```python
from build123d import *

# Parameters (mm, degrees)
SKETCH_1_W          = 104
SKETCH_1_H          = 52
SKETCH_1_R          = 11.25
EXTRUDE_1_DEPTH     = 6
SKETCH_2_R          = 2.15
SKETCH_2_R_2        = 5
CUT_EXTRUDE_1_DEPTH = 10
FILLET_2_R          = 5
SKETCH_3_R          = 1.6
SKETCH_3_R_2        = 2.1
CUT_EXTRUDE_2_DEPTH = 10
SKETCH1_R           = 4
CUT_EXTRUDE1_DEPTH  = 2


with BuildPart() as part:
    # 草图1 → 凸台-拉伸1 (new body)
    with BuildSketch(Plane(origin=(0, 0, 0), x_dir=(0, 0, -1), z_dir=(1, 0, 0))):
        with Locations((245.135135135, 41.033128111)):
            Rectangle(SKETCH_1_W, SKETCH_1_H)
        with Locations((220.135135135, 41.033128111)):
            Circle(SKETCH_1_R, mode=Mode.SUBTRACT)
        with Locations((270.135135135, 41.033128111)):
            Circle(SKETCH_1_R, mode=Mode.SUBTRACT)
    extrude(amount=EXTRUDE_1_DEPTH)

    # 草图2 → 切除-拉伸1 (cut)
    # profile 1 of 12: a face of its own
    with BuildSketch(Plane(origin=(6, 0, 0), x_dir=(0, 0, -1), z_dir=(1, 0, 0))):
        with Locations((198.135135135, 62.033128111)):
            Circle(SKETCH_2_R)
    # profile 2 of 12: a face of its own
    with BuildSketch(Plane(origin=(6, 0, 0), x_dir=(0, 0, -1), z_dir=(1, 0, 0))):
        with Locations((198.135135135, 20.033128111)):
            Circle(SKETCH_2_R)
    # profile 3 of 12: a face of its own
    with BuildSketch(Plane(origin=(6, 0, 0), x_dir=(0, 0, -1), z_dir=(1, 0, 0))):
        with Locations((245.135135135, 20.033128111)):
            Circle(SKETCH_2_R_2)
        with Locations((245.135135135, 20.033128111)):
            Circle(SKETCH_2_R, mode=Mode.SUBTRACT)
    # profile 4 of 12: a face of its own
    with BuildSketch(Plane(origin=(6, 0, 0), x_dir=(0, 0, -1), z_dir=(1, 0, 0))):
        with BuildLine():
            Line((245.13513516, 15.033128111), (250.135135135, 15.033128111))
            Line((250.135135135, 15.033128111), (250.135135135, 20.033128111))
            ThreePointArc((250.135135135, 20.033128111), (248.67066905, 16.497594214), (245.13513516, 15.033128111))
        make_face()
    # profile 5 of 12: a face of its own
    with BuildSketch(Plane(origin=(6, 0, 0), x_dir=(0, 0, -1), z_dir=(1, 0, 0))):
        with BuildLine():
            Line((240.135135135, 15.033128111), (245.13513516, 15.033128111))
            ThreePointArc((245.13513516, 15.033128111), (241.599601238, 16.497594196), (240.135135135, 20.033128111))
            Line((240.135135135, 20.033128111), (240.135135135, 15.033128111))
        make_face()
    # profile 6 of 12: a face of its own
    with BuildSketch(Plane(origin=(6, 0, 0), x_dir=(0, 0, -1), z_dir=(1, 0, 0))):
        with Locations((245.135135135, 20.033128111)):
            Circle(SKETCH_2_R)
    # profile 7 of 12: a face of its own
    with BuildSketch(Plane(origin=(6, 0, 0), x_dir=(0, 0, -1), z_dir=(1, 0, 0))):
        with Locations((245.135135135, 62.033128111)):
            Circle(SKETCH_2_R_2)
        with Locations((245.135135135, 62.033128111)):
            Circle(SKETCH_2_R, mode=Mode.SUBTRACT)
    # profile 8 of 12: a face of its own
    with BuildSketch(Plane(origin=(6, 0, 0), x_dir=(0, 0, -1), z_dir=(1, 0, 0))):
        with Locations((245.135135135, 62.033128111)):
            Circle(SKETCH_2_R)
    # profile 9 of 12: a face of its own
    with BuildSketch(Plane(origin=(6, 0, 0), x_dir=(0, 0, -1), z_dir=(1, 0, 0))):
        with BuildLine():
            ThreePointArc((245.135135095, 67.033128111), (248.670669027, 65.568662031), (250.135135135, 62.033128111))
            Line((250.135135135, 62.033128111), (250.135135135, 67.033128111))
            Line((250.135135135, 67.033128111), (245.135135095, 67.033128111))
        make_face()
    # profile 10 of 12: a face of its own
    with BuildSketch(Plane(origin=(6, 0, 0), x_dir=(0, 0, -1), z_dir=(1, 0, 0))):
        with BuildLine():
            Line((240.135135135, 67.033128111), (240.135135135, 62.033128111))
            ThreePointArc((240.135135135, 62.033128111), (241.599601215, 65.568662003), (245.135135095, 67.033128111))
            Line((245.135135095, 67.033128111), (240.135135135, 67.033128111))
        make_face()
    # profile 11 of 12: a face of its own
    with BuildSketch(Plane(origin=(6, 0, 0), x_dir=(0, 0, -1), z_dir=(1, 0, 0))):
        with Locations((292.135135135, 62.033128111)):
            Circle(SKETCH_2_R)
    # profile 12 of 12: a face of its own
    with BuildSketch(Plane(origin=(6, 0, 0), x_dir=(0, 0, -1), z_dir=(1, 0, 0))):
        with Locations((292.135135135, 20.033128111)):
            Circle(SKETCH_2_R)
    extrude(amount=-CUT_EXTRUDE_1_DEPTH, mode=Mode.SUBTRACT)

    # 圆角2
    fillet_2_edges = [part.edges().sort_by_distance(p)[0] for p in [
        (3, 15.033128111, -240.135135135),
        (3, 15.033128111, -193.135135135),
        (3, 67.033128111, -240.135135135),
        (3, 67.033128111, -250.135135135),
        (3, 67.033128111, -297.135135135),
        (3, 15.033128111, -297.135135135),
        (3, 15.033128111, -250.135135135),
        (3, 67.033128111, -193.135135135),
    ]]
    fillet(fillet_2_edges, radius=FILLET_2_R - 0.0001)  # a hair under: the kernel refuses the full size

    # 草图3 → 切除-拉伸2 (cut)
    with BuildSketch(Plane(origin=(6, 0, 0), x_dir=(0, 0, -1), z_dir=(1, 0, 0))):
        with Locations((220.135135135, 55.033128111)):
            Circle(SKETCH_3_R)
        with Locations((228.135135135, 54.889534571)):
            Circle(SKETCH_3_R_2)
        with Locations((228.135135135, 27.17672165)):
            Circle(SKETCH_3_R_2)
        with Locations((212.135135135, 27.17672165)):
            Circle(SKETCH_3_R_2)
        with Locations((212.135135135, 54.889534571)):
            Circle(SKETCH_3_R_2)
        with Locations((234.135135135, 41.033128111)):
            Circle(SKETCH_3_R)
        with Locations((220.135135135, 27.033128111)):
            Circle(SKETCH_3_R)
        with Locations((206.135135135, 41.033128111)):
            Circle(SKETCH_3_R)
        with Locations((284.135135135, 41.033128111)):
            Circle(SKETCH_3_R)
        with Locations((270.135135135, 27.033128111)):
            Circle(SKETCH_3_R)
        with Locations((256.135135135, 41.033128111)):
            Circle(SKETCH_3_R)
        with Locations((278.135135135, 54.889534571)):
            Circle(SKETCH_3_R_2)
        with Locations((278.135135135, 27.17672165)):
            Circle(SKETCH_3_R_2)
        with Locations((262.135135135, 27.17672165)):
            Circle(SKETCH_3_R_2)
        with Locations((262.135135135, 54.889534571)):
            Circle(SKETCH_3_R_2)
        with Locations((270.135135135, 55.033128111)):
            Circle(SKETCH_3_R)
    extrude(amount=-CUT_EXTRUDE_2_DEPTH, mode=Mode.SUBTRACT)

    # Sketch1 → Cut-Extrude1 (cut)
    with BuildSketch(Plane.ZY):
        with Locations((-278.135135135, 27.17672165)):
            Circle(SKETCH1_R)
        with Locations((-278.135135135, 54.889534571)):
            Circle(SKETCH1_R)
        with Locations((-262.135135135, 54.889534571)):
            Circle(SKETCH1_R)
        with Locations((-262.135135135, 27.17672165)):
            Circle(SKETCH1_R)
        with Locations((-228.135135135, 54.889534571)):
            Circle(SKETCH1_R)
        with Locations((-212.135135135, 54.889534571)):
            Circle(SKETCH1_R)
        with Locations((-212.135135135, 27.17672165)):
            Circle(SKETCH1_R)
        with Locations((-228.135135135, 27.17672165)):
            Circle(SKETCH1_R)
    extrude(amount=-CUT_EXTRUDE1_DEPTH, mode=Mode.SUBTRACT)


solid = part.part
```
Check sheet for the modelled part. Datum: model origin and axes. Units: mm. A direction names the side the tool comes from. Give positions to 0.01 mm unless a question says otherwise; leave off trailing zeros. Loops run counter-clockwise (first coordinate to the right, second up) from the corner with the lowest first, then second, coordinate; pieces in that order, holes last. Notation, with made-up numbers: M 86,3 L 111,3 A12 cw 111,12 Z; hole C 10,32.25 d9. An arc over 180 degrees is marked long. Answer in a Markdown table with one row per item.
1) Depth check by flat-ended pin: pin 1 (2.5 mm diameter, centred on y = 54.89, z = -262.14, fed in from +X); pin 2 (6.5 mm diameter, centred on y = 56, z = -278.5, fed in from -X). Enter the tip coordinate at first touch or a pass-through.
Solutions:
| item | result |
|---|---|
| pin 1 | passes through |
| pin 2 | stops at x = 0 |
2) Cross-section at A-A (z = -279). Enter the section's corners in (x, y).
Solutions:
| item | result |
|---|---|
| outline | M 0,15.03 L 6,15.03 L 6,25.26 L 2,25.26 L 2,23.27 L 0,23.27 Z; M 0,31.08 L 2,31.08 L 2,29.09 L 6,29.09 L 6,34.11 L 0,34.11 Z; M 0,47.96 L 6,47.96 L 6,52.98 L 2,52.98 L 2,50.98 L 0,50.98 Z; M 0,58.79 L 2,58.79 L 2,56.8 L 6,56.8 L 6,67.03 L 0,67.03 Z |
3) Thickness scan on line 1 (Y direction, x = 1.35, z = -292); line 2 (Z direction, x = 3.9, y = 48); line 3 (Z direction, x = 0.5, y = 20.5). Record the ranges inside material, lowest first.
Solutions:
| item | result |
|---|---|
| line 1 | y = 15.03 to 17.89, 22.18 to 59.89, 64.18 to 67.03 |
| line 2 | z = -297.14 to -278.97, -261.3 to -228.97, -211.3 to -193.14 |
| line 3 | z = -297.14 to -294.23, -290.04 to -250.11, -240.16 to -200.23, -196.04 to -193.14 |
4) Cross-section at B-B (y = 47). Enter the section's corners in (x, z), plus the area to 3 significant figures.
Solutions:
| item | result |
|---|---|
| outline | M 0,-297.14 L 6,-297.14 L 6,-279.67 L 0,-279.67 Z; M 0,-260.6 L 6,-260.6 L 6,-229.67 L 0,-229.67 Z; M 0,-210.6 L 6,-210.6 L 6,-193.14 L 0,-193.14 Z |
| area | 395 mm^2 |
5) Cross-section at D-D (x = 3.1). Count the separate pieces of the cut face and the enclosed holes in it, plus the area to 3 significant figures.
Solutions:
| item | result |
|---|---|
| separate pieces | 1 |
| enclosed holes | 22 |
| area | 4,160 mm^2 |
6) Tool access check on faces 1 (the face through (4.028, 26.372, -214.075)), 2 (the face through (2.96, 65.53, -251.56)), 3 (the face through (0.99, 25.64, -274.44)). Record the directions out of +Z, -Z, +X, -X, +Y, -Y that give a thin tool (end or side, any length) a straight path to the whole face; none if there is none.
Solutions:
| item | result |
|---|---|
| face 1 | +X, -X |
| face 2 | +X, -X, +Y |
| face 3 | -X |
7) Cross-section at C-C (z = -206.5). Enter the section's corners in (x, y), plus the area to 3 significant figures.
Solutions:
| item | result |
|---|---|
| outline | M 0,15.03 L 6,15.03 L 6,39.48 L 0,39.48 Z; M 0,42.59 L 6,42.59 L 6,67.03 L 0,67.03 Z |
| area | 293 mm^2 |
8) Mould release check, pull along Y, two halves, no side actions. Record for faces 4 (the face through (3.04, 65.53, -194.56)), 5 (the face through (0, 41, -244)), 6 (the face through (3.04, 25.03, -245.25)), 7 (the face through (3.04, 39.47, -205.79)): released by +Y, released by -Y, zero draft, split by the parting line, or undercut.
Solutions:
| item | result |
|---|---|
| face 4 | released by +Y |
| face 5 | zero draft |
| face 6 | released by -Y |
| face 7 | undercut |
